Check sheet for the modelled part. Datum: model origin and axes. Units: mm. A direction names the side the tool comes from. Round coordinates to 2 decimals unless told otherwise and drop trailing zeros. Order: outer loops, then holes, each group sorted by start corner. A loop starts at its lowest first (then second) coordinate and runs counter-clockwise, first axis right, second up. Notation, with made-up numbers: (45, 10) -> (50, 10) arc R15 cw to (50, 32) -> close; hole circle Ø8 at (35.5, 62). An arc over 180 degrees is marked (long way). Answer in a Markdown table with one row per item.
from build123d import *

# Parameters (mm, degrees)
SKETCH11_W                     = 3.4
SKETCH11_H                     = 62.2
BASE_FLANGE3_DEPTH             = 30
EDGE_FLANGE1_STRIP_W           = 15.1
EDGE_FLANGE1_STRIP_H           = 3.4
EDGE_FLANGE1_STRIP_CUT_DEPTH   = 30
EDGE_FLANGE1_STRIP_2_W         = 15.1
EDGE_FLANGE1_STRIP_2_H         = 3.4
EDGE_FLANGE1_STRIP_CUT_2_DEPTH = 30
EDGE_FLANGE1_DEPTH             = 30
EDGE_FLANGE1_BEND_DEPTH        = 30
SKETCH22_R                     = 1.5
CUT_EXTRUDE1_DEPTH             = 72.894645141


# Sheet-metal steps are written as plain solids
with BuildPart() as part:
    # Sketch11 → Base-Flange3 (new body)
    with BuildSketch(Plane.XY):
        with Locations((-1.7, 0)):
            Rectangle(SKETCH11_W, SKETCH11_H)
    extrude(amount=BASE_FLANGE3_DEPTH)

    # Edge-Flange1 strip (across the edge) → Edge-Flange1 strip cut (cut)
    with BuildSketch(Plane(origin=(-3.4, 31.1, 30), x_dir=(0, -1, 0), z_dir=(0, 0, -1))):
        with Locations((-3.4, -1.7)):
            Rectangle(EDGE_FLANGE1_STRIP_W, EDGE_FLANGE1_STRIP_H)
    extrude(amount=EDGE_FLANGE1_STRIP_CUT_DEPTH, mode=Mode.SUBTRACT)

    # Edge-Flange1 strip 2 (across the edge) → Edge-Flange1 strip cut 2 (cut)
    with BuildSketch(Plane(origin=(-3.4, -31.1, 0), x_dir=(0, 1, 0), z_dir=(0, 0, 1))):
        with Locations((-3.4, -1.7)):
            Rectangle(EDGE_FLANGE1_STRIP_2_W, EDGE_FLANGE1_STRIP_2_H)
    extrude(amount=EDGE_FLANGE1_STRIP_CUT_2_DEPTH, mode=Mode.SUBTRACT)

    # Edge-Flange1 section (across the edge) → Edge-Flange1 (add)
    with BuildSketch(Plane(origin=(-3.4, 31.1, 30), x_dir=(0, -1, 0), z_dir=(0, 0, -1))):
        with BuildLine():
            Line((0, 0.75), (0, 16.6))
            Line((0, 16.6), (3.4, 16.6))
            Line((3.4, 16.6), (3.4, 0.75))
            ThreePointArc((3.4, 0.75), (3.619669914, 0.219669914), (4.15, 0))
            Line((4.15, 0), (4.15, -3.4))
            ThreePointArc((4.15, -3.4), (1.215506858, -2.184493142), (0, 0.75))
        make_face()
    extrude(amount=EDGE_FLANGE1_DEPTH)

    # Edge-Flange1 section 2 (across the edge) → Edge-Flange1 bend (add)
    with BuildSketch(Plane(origin=(-3.4, -31.1, 0), x_dir=(0, 1, 0), z_dir=(0, 0, 1))):
        with BuildLine():
            Line((0, 0.75), (0, 16.6))
            Line((0, 16.6), (3.4, 16.6))
            Line((3.4, 16.6), (3.4, 0.75))
            ThreePointArc((3.4, 0.75), (3.619669914, 0.219669914), (4.15, 0))
            Line((4.15, 0), (4.15, -3.4))
            ThreePointArc((4.15, -3.4), (1.215506858, -2.184493142), (0, 0.75))
        make_face()
    extrude(amount=EDGE_FLANGE1_BEND_DEPTH)

    # Sketch22 → Cut-Extrude1 (cut, through all)
    with BuildSketch(Plane(origin=(0, 31.1, 0), x_dir=(1, 0, 0), z_dir=(0, 1, 0))):
        with Locations(Location((-12.329371406, -23.693332437, 0), (0, 0, 180))):
            Circle(SKETCH22_R)
        with Locations(Location((-12.329371406, -6.306667563, 0), (0, 0, 180))):
            Circle(SKETCH22_R)
    extrude(amount=-CUT_EXTRUDE1_DEPTH, mode=Mode.SUBTRACT)


solid = part.part
Item 1: Cross-section at A-A (x = -6.5). Record the boundary of the cut face in (y, z).
Result sheet:
| item | result |
|---|---|
| outline | (-31.1, 0) -> (-27.7, 0) -> (-27.7, 30) -> (-31.1, 30) -> close; (27.7, 0) -> (31.1, 0) -> (31.1, 30) -> (27.7, 30) -> close |
Item 2: Scan lines: line 1 (Y direction, x = -16.75, z = 11.75); line 2 (X direction, y = -14.5, z = 4); line 3 (Y direction, x = -2.5, z = 8). Record each from-to range of solid material in increasing order. Write a range as [from, to].
Result sheet:
| item | result |
|---|---|
| line 1 | y = [-31.1, -27.7], [27.7, 31.1] |
| line 2 | x = [-3.4, 0] |
| line 3 | y = [-30.76, 30.76] |
Item 3: Mould release check, pull along X, two halves, no side actions. Record for faces 3 (the flat face through (-12, -27.7, 15)), 4 (the cylindrical face through (-1.18, -29.85, 14.79)), 5 (the cylindrical face through (-13.76, -29.38, 24.14)), 6 (the cylindrical face through (-13.7, -29.4, 5.7)): pulls with the +X half, pulls with the -X half, needs draft (parallel to the pull), parting line crosses it, or undercut.
Result sheet:
| item | result |
|---|---|
| face 3 | needs draft |
| face 4 | pulls with the +X half |
| face 5 | undercut |
| face 6 | undercut |
Item 4: Set-up check for faces 1 (the cylindrical face through (-13.7, 29.4, 5.7)), 2 (the flat face through (-12, 27.7, 15)): record each of +Z, -Z, +X, -X, +Y, -Y from which the full face is reachable in a straight line by a thin tool's end or side.
Result sheet:
| item | result |
|---|---|
| face 1 | +Y, -Y |
| face 2 | +Z, -Z, -X |
Item 5: Cross-section at C-C (y = -13). Record the boundary of the cut face in (x, z).
Result sheet:
| item | result |
|---|---|
| outline | (-3.4, 0) -> (0, 0) -> (0, 30) -> (-3.4, 30) -> close |
Item 6: Cross-section at B-B (z = 11.25). Record the boundary of the cut face in (x, y).
Result sheet:
| item | result |
|---|---|
| outline | (-20, -31.1) -> (-4.15, -31.1) arc R4.15 ccw to (0, -26.95) -> (0, 26.95) arc R4.15 ccw to (-4.15, 31.1) -> (-20, 31.1) -> (-20, 27.7) -> (-4.15, 27.7) arc R0.75 cw to (-3.4, 26.95) -> (-3.4, -26.95) arc R0.75 cw to (-4.15, -27.7) -> (-20, -27.7) -> close |
Item 7: Cross-section at D-D (x = -2). Record the boundary of the cut face in (y, z).
Result sheet:
| item | result |
|---|---|
| outline | (-30.5, 0) -> (30.5, 0) -> (30.5, 30) -> (-30.5, 30) -> close |
Item 8: Depth check by flat-ended pin: P1, Ø12, axis at y = 21, z = 20.5, coming from the -X side; P2, Ø3.5, axis at x = -12.33, z = 23.69, coming from the +Y side. Enter the tip coordinate at first touch or a pass-through.
Result sheet:
| item | result |
|---|---|
| P1 | stops at x = -3.4 |
| P2 | stops at y = 31.1 |
